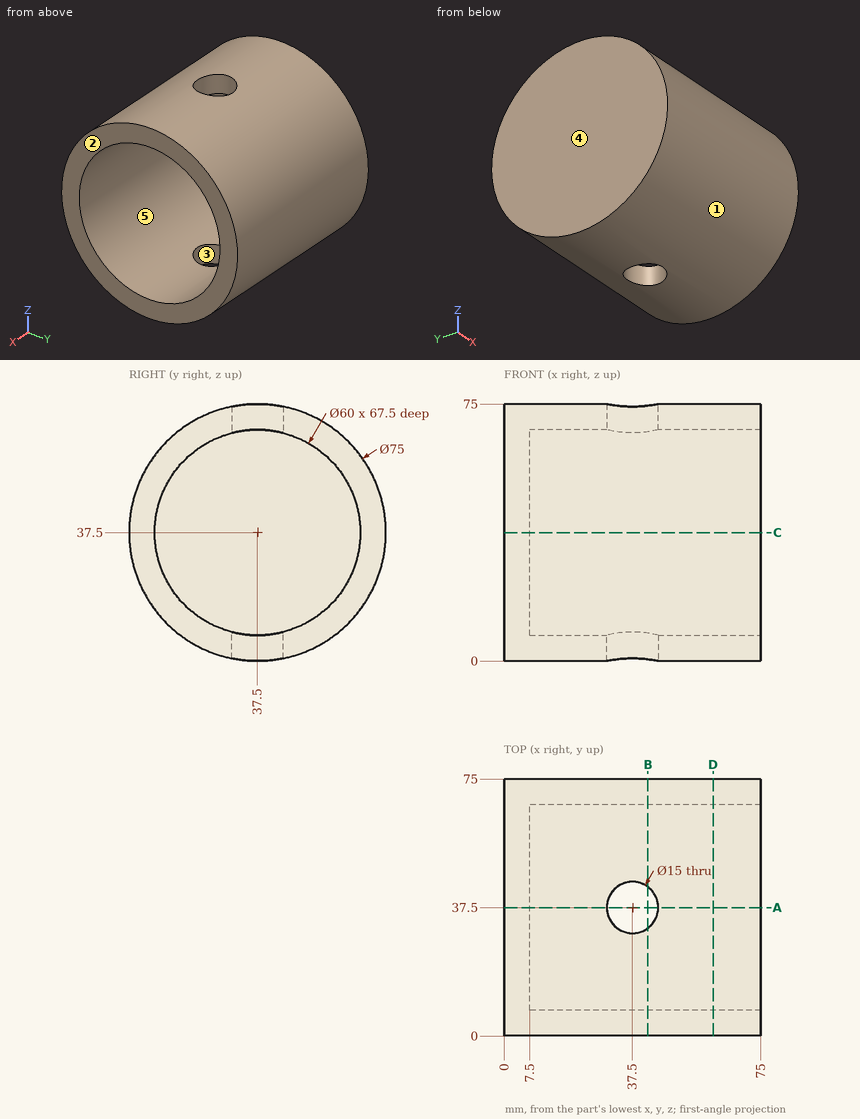
Answer from the drawing. Dimensions are ordinates in mm from the lowest x, y and z of the part. A direction names the side the tool comes from. Coordinates: 2 decimals unless noted, no trailing zeros. Loops run counter-clockwise (first coordinate to the right, second up) from the corner with the lowest first, then second, coordinate; pieces in that order, holes last.
Q1. The mould has two halves that part along Y. Classify the marked faces 1, 2 and 3: +Y half, -Y half, draft (parallel to the pull), parting line (faces both ways), or undercut.
Q2. Consider probe 1 along Z at (x, y) = (10, 36.5); probe 2 along X at (y, z) = (37, 4); probe 3 along Y at (x, z) = (47, 37.5). Determine where each line is inside the solid, lowest interval first.
Q3. The part is cut by section C-C on z = 37.5. Write down the section's boundary in (x, y).
Q4. The part is cut by section B-B on x = 42. Write down the section's boundary in (y, z), and give its area (3 significant figures).
Q5. The part is cut by section D-D on x = 61. Write down the section's boundary in (y, z).
Q6. Which of the six approach directions +Z, -Z, +X, -X, +Y, -Y give full straight-line access (tool end or side, diameter ignored) to the marked faces 4 and 5?
Q7. The part is cut by section A-A on y = 37.5. Write down the section's boundary in (x, z), and give its area (3 significant figures).
Q8. Each of these flat-tipped pins is pushed along its axis until it touches: pin 1 Ø1.5 at (x, z) = (28.5, 58.5) entering from +Y; pin 2 Ø13.5 at (x, y) = (37.5, 37.5) entering from +Z; pin 3 Ø12 at (x, z) = (58, 63) entering from -Y; pin 4 Ø3 at (y, z) = (52.5, 48.5) entering from +X. Where does it stop, or does it pass through?
Results below:
1. face 1: parting line
1. face 2: draft
1. face 3: undercut
2. probe 1: z = 0.01 to 7.52, 67.48 to 74.99
2. probe 2: x = 0 to 30.02, 44.98 to 75
2. probe 3: y = 0 to 7.5, 67.5 to 75
3. outline: (0, 0) - (75, 0) - (75, 7.5) - (7.5, 7.5) - (7.5, 67.5) - (75, 67.5) - (75, 75) - (0, 75) - close
4. outline: (31.5, 0.48) - (31.5, 8.11) arc R30 cw to (31.5, 66.89) - (31.5, 74.52) arc R37.5 ccw to start; (43.5, 0.48) arc R37.5 ccw to (43.5, 74.52) - (43.5, 66.89) arc R30 cw to (43.5, 8.11) - close
4. area: 1,410 mm2
5. outline: circle Ø75 at (37.5, 37.5); hole circle Ø60 at (37.5, 37.5)
6. face 4: +Z, -Z, -X, +Y, -Y
6. face 5: +X
7. outline: (0, 0) - (30, 0) - (30, 7.5) - (7.5, 7.5) - (7.5, 67.5) - (30, 67.5) - (30, 75) - (0, 75) - close; (45, 0) - (75, 0) - (75, 7.5) - (45, 7.5) - close; (45, 67.5) - (75, 67.5) - (75, 75) - (45, 75) - close
7. area: 1,350 mm2
8. pin 1: stops at y = 69.06
8. pin 2: passes through
8. pin 3: stops at y = 5.47
8. pin 4: stops at x = 7.5
